Here's how the part is built. I have some questions about the finished solid (model axes, mm). A direction names the side the tool comes from. Give positions to 0.01 mm unless a question says otherwise; leave off trailing zeros. Loops run counter-clockwise (first coordinate to the right, second up) from the corner with the lowest first, then second, coordinate; pieces in that order, holes last. Notation, with made-up numbers: (88.25, -37.75) -> (137.25, -37.75) arc R17 ccw to (137.25, -13.75) -> close; hole circle Ø5 at (19, 78.25). An arc over 180 degrees is marked (long way). Answer in a Markdown table with one row per item. Add a question column.
Item 1: If we section it at C-C (z = 28): Write out the boundary of the cut face in (x, y).
Item 2: For P1, Ø6, axis at x = -107.5, y = 2.5, coming from the +Z side; P2, Ø5, axis at x = 50, y = -3.5, coming from the +Z side; P3, Ø17.5, axis at x = -59.5, z = -14, coming from the +Y side; P4, Ø4, axis at x = 111, y = 5.1, coming from the +Z side, each with a flat end and sliding along its axis, tell me the tip position at first contact or that it passes through.
Item 3: If we section it at B-B (x = -60): Write out the boundary of the cut face in (y, z), then the cut area to 3 significant figures.
Item 4: If we section it at D-D (z = -15): Give the number of separate pieces and of enclosed holes in the cut face, then the cut area to 3 significant figures.
Item 5: We'd pull the mould along Z, two halves only. Please class faces 6 (the face through (-48, -13, -11)), 7 (the face through (110.662, 10.877, 46.735)), 8 (the face through (62.003, -12.714, -14.369)): released by +Z, released by -Z, zero draft, split by the parting line, or undercut.
Item 6: If I drill on line 1 (X direction, y = -10.25, z = 57); line 2 (Z direction, x = 60, y = -15); line 3 (X direction, y = -9.5, z = -16.5), over which ranges is the centre line in solid material (lowest first)?
Item 7: Which directions (+Z, -Z, +X, -X, +Y, -Y) give clear straight access to the entire face, cutting with the end or side of a thin tool? Please do faces 1 (the face through (-107.4, 5, 49)), 2 (the face through (-1, -14.7, 5)), 3 (the face through (-60, -8.7, -10)), 4 (the face through (38, -4, 11.43)), 5 (the face through (62, -13.7, -17)).
Item 8: If we section it at A-A (z = 59): Write out the boundary of the cut face in (x, y).
```python
from build123d import *

# Parameters (mm, degrees)
F1_DEPTH  = 8
F3_DEPTH  = 1.9
F5_DEPTH  = 2.5
F7_DEPTH  = 2.3
F9_W      = 14
F9_H      = 22
F10_DEPTH = 12
F11_DEPTH = 2
F12_W     = 12.1
F12_H     = 20
F13_W     = 12.1
F13_H     = 20
F14_DEPTH = 2
F17_R     = 5.99999
F18_R     = 5.99999
F19_DEPTH = 10
F20_DEPTH = 25
F22_R     = 2.1
F21_R     = 2.1
F23_DEPTH = 10
F24_SIZE  = 1.5
F25_W     = 24
F25_H     = 8
F26_DEPTH = 28
F28_R     = 4.1
F27_R     = 4.1
F29_DEPTH = 3
F30_R     = 2.1
F31_DEPTH = 28.701
F32_R     = 3.6
F33_DEPTH = 3
F34_R     = 5
F35_W     = 20
F35_H     = 8
F36_DEPTH = 5
F37_SIZE  = 1
F38_W     = 27
F38_H     = 8
F39_DEPTH = 2


# Not quite as in the source:
# - a fillet or chamfer is up to 0.001 mm smaller than in the source, because OpenCascade refuses the exact size
# - a feature names something its author has since deleted; it is built from what else it names


with BuildPart() as f1:
    # F0 (on Front) → F1 (new body)
    with BuildSketch(Plane.XZ):
        Polygon((-118.5, 0), (118.5, 0), (118.5, 66.23), (104.5, 66.23), (104.5, 13.43), (-104.5, 13.43), (-104.5, 66.23), (-118.5, 66.23), align=None)
    extrude(amount=F1_DEPTH)

    # F2 (on face) → F3 (join)
    with BuildSketch(Plane.XZ.offset(8)):
        Polygon((-116.6, 66.23), (-118.5, 66.23), (-118.5, 0), (118.5, 0), (118.5, 66.23), (116.6, 66.23), (116.6, 3.43), (-116.6, 3.43), align=None)
    extrude(amount=F3_DEPTH)

    # F4 (on face) → F5 (join)
    with BuildSketch(Plane.XZ.offset(9.9)):
        Polygon((-113.5, 66.23), (-118.5, 66.23), (-118.5, 0), (118.5, 0), (118.5, 66.23), (113.5, 66.23), (113.5, 8), (-113.5, 8), align=None)
    extrude(amount=F5_DEPTH)

    # F6 (on face) → F7 (join)
    with BuildSketch(Plane.XZ.offset(12.4)):
        Polygon((-116.6, 66.23), (-118.5, 66.23), (-118.5, 0), (118.5, 0), (118.5, 66.23), (116.6, 66.23), (116.6, 3.43), (-116.6, 3.43), align=None)
    extrude(amount=F7_DEPTH)

    # F9 (on face) → F10 (join)
    with BuildSketch(Plane(origin=(0, 0, 0), x_dir=(-1, 0, 0), z_dir=(0, 1, 0))):
        with Locations((111.5, 55.23)):
            Rectangle(F9_W, F9_H)
        with Locations((-111.5, 55.23)):
            Rectangle(F9_W, F9_H)
    extrude(amount=F10_DEPTH)

    # F8 (on face) → F11 (join)
    with BuildSketch(Plane.XZ.offset(14.7)):
        Polygon((-111.5, 66.23), (-118.5, 66.23), (-118.5, 0), (118.5, 0), (118.5, 66.23), (111.5, 66.23), (111.5, 7), (-111.5, 7), align=None)
    extrude(amount=F11_DEPTH)

    # F12 (on face) + F13 (on face) → F14 (cut)
    with BuildSketch(Plane.XY.offset(66.23)):
        with Locations((-110.55, 2)):
            Rectangle(F12_W, F12_H)
    with BuildSketch(Plane.XY.offset(66.23)):
        with Locations((110.55, 2)):
            Rectangle(F13_W, F13_H)
    extrude(amount=-F14_DEPTH, mode=Mode.SUBTRACT)

    # F17 (radius 6 in the source; OpenCascade refuses exactly that, so slightly less here)
    f17_edges = [f1.edges().sort_by_distance(p)[0] for p in [
        (-111.5, 0, 44.23),
        (-111.5, 12, 44.23),
    ]]
    fillet(f17_edges, radius=F17_R)

    # F18 (radius 6 in the source; OpenCascade refuses exactly that, so slightly less here)
    f18_edges = [f1.edges().sort_by_distance(p)[0] for p in [
        (111.5, 0, 44.23),
        (111.5, 12, 44.23),
    ]]
    fillet(f18_edges, radius=F18_R)

    # F15 (on face) + F16 (on face) → F19 (cut)
    with BuildSketch(Plane(origin=(0, 0, 44.23), x_dir=(1, 0, 0), z_dir=(0, 0, -1))):
        Polygon((111, -1.1430780618), (107.4, -3.2215390309), (107.4, -7.3784609691), (111, -9.4569219382), (114.6, -7.3784609691), (114.6, -3.2215390309), align=None)
    with BuildSketch(Plane(origin=(0, 0, 44.23), x_dir=(1, 0, 0), z_dir=(0, 0, -1))):
        Polygon((-107.4, -7.3784609691), (-107.4, -3.2215390309), (-111, -1.1430780618), (-114.6, -3.2215390309), (-114.6, -7.3784609691), (-111, -9.4569219382), align=None)
    extrude(amount=-F19_DEPTH, mode=Mode.SUBTRACT)

    # F15 (on face) + F16 (on face) → F20 (cut)
    with BuildSketch(Plane(origin=(0, 0, 44.23), x_dir=(1, 0, 0), z_dir=(0, 0, -1))):
        Polygon((111, -1.1430780618), (107.4, -3.2215390309), (107.4, -7.3784609691), (111, -9.4569219382), (114.6, -7.3784609691), (114.6, -3.2215390309), align=None)
    with BuildSketch(Plane(origin=(0, 0, 44.23), x_dir=(1, 0, 0), z_dir=(0, 0, -1))):
        Polygon((-107.4, -7.3784609691), (-107.4, -3.2215390309), (-111, -1.1430780618), (-114.6, -3.2215390309), (-114.6, -7.3784609691), (-111, -9.4569219382), align=None)
    extrude(amount=F20_DEPTH, mode=Mode.SUBTRACT)

    # F22 (on face) + F21 (on face) → F23 (cut, through all)
    with BuildSketch(Plane.XY.offset(64.23)):
        with Locations((111, 5.1)):
            Circle(F22_R)
    with BuildSketch(Plane.XY.offset(64.23)):
        with Locations((-111, 5.1)):
            Circle(F21_R)
    extrude(amount=-F23_DEPTH, mode=Mode.SUBTRACT)

    # F24
    f24_edges = [f1.edges().sort_by_distance(p)[0] for p in [
        (118.5, 0, 19.115005),
        (-118.5, 0, 19.115005),
        (0, 0, 0),
        (118.5, 12, 58.229995),
        (118.5, 10.242644, 45.987356),
        (118.5, 6, 44.23),
        (118.5, 1.757356, 42.472644),
        (-118.5, 1.757356, 42.472644),
        (-118.5, 6, 44.23),
        (-118.5, 10.242644, 45.987356),
        (-118.5, 12, 58.229995),
    ]]
    chamfer(f24_edges, length=F24_SIZE)

    # F25 (on face) → F26 (join)
    with BuildSketch(Plane(origin=(0, 0, 0), x_dir=(1, 0, 0), z_dir=(0, 0, -1))):
        with Locations((-60, 12.7)):
            Rectangle(F25_W, F25_H)
        with Locations((60, 12.7)):
            Rectangle(F25_W, F25_H)
    extrude(amount=F26_DEPTH)

    # F28 (on face) + F27 (on face) → F29 (cut)
    with BuildSketch(Plane(origin=(0, -8.7, 0), x_dir=(-1, 0, 0), z_dir=(0, 1, 0))):
        with Locations((-60, -15)):
            Circle(F28_R)
    with BuildSketch(Plane(origin=(0, -8.7, 0), x_dir=(-1, 0, 0), z_dir=(0, 1, 0))):
        with Locations((60, -15)):
            Circle(F27_R)
    extrude(amount=-F29_DEPTH, mode=Mode.SUBTRACT)

    # F30 (on face) → F31 (cut, through all)
    with BuildSketch(Plane.XZ.offset(16.7)):
        with Locations((-60, -15)):
            Circle(F30_R)
        with Locations((60, -15)):
            Circle(F30_R)
    extrude(amount=-F31_DEPTH, mode=Mode.SUBTRACT)

    # F32 (on face) → F33 (cut)
    with BuildSketch(Plane.XZ.offset(16.7)):
        with Locations((-60, -15)):
            Circle(F32_R)
        with Locations((60, -15)):
            Circle(F32_R)
    extrude(amount=-F33_DEPTH, mode=Mode.SUBTRACT)

    # F34
    f34_edges = [f1.edges().sort_by_distance(p)[0] for p in [
        (-72, -12.7, -28),
        (-48, -12.7, -28),
        (48, -12.7, -28),
        (72, -12.7, -28),
    ]]
    fillet(f34_edges, radius=F34_R)

    # F35 (on face) → F36 (cut)
    with BuildSketch(Plane.XY.offset(13.43)):
        with Locations((-21.5, -4)):
            Rectangle(F35_W, F35_H)
    extrude(amount=-F36_DEPTH, mode=Mode.SUBTRACT)

    # F37
    f37_edges = [f1.edges().sort_by_distance(p)[0] for p in [
        (-72, -8.7, -11.5),
        (72, -8.7, -11.5),
        (48, -8.7, -11.5),
        (-48, -8.7, -11.5),
        (-70.535534, -8.7, -26.535534),
        (-60, -8.7, -28),
        (-49.464466, -8.7, -26.535534),
        (49.464466, -8.7, -26.535534),
        (60, -8.7, -28),
        (70.535534, -8.7, -26.535534),
    ]]
    chamfer(f37_edges, length=F37_SIZE)

    # F38 (on face) → F39 (cut)
    with BuildSketch(Plane.XY.offset(13.43)):
        with Locations((38.1, -4)):
            Rectangle(F38_W, F38_H)
    extrude(amount=-F39_DEPTH, mode=Mode.SUBTRACT)


solid = f1.part
```
Recorded:
| question | item | result |
|---|---|---|
| 1 | outline | (-118.5, -16.7) -> (-111.5, -16.7) -> (-111.5, -14.7) -> (-116.6, -14.7) -> (-116.6, -12.4) -> (-113.5, -12.4) -> (-113.5, -9.9) -> (-116.6, -9.9) -> (-116.6, -8) -> (-104.5, -8) -> (-104.5, 0) -> (-117, 0) -> (-118.5, -1.5) -> close; (104.5, -8) -> (116.6, -8) -> (116.6, -9.9) -> (113.5, -9.9) -> (113.5, -12.4) -> (116.6, -12.4) -> (116.6, -14.7) -> (111.5, -14.7) -> (111.5, -16.7) -> (118.5, -16.7) -> (118.5, -1.5) -> (117, 0) -> (104.5, 0) -> close |
| 2 | P1 | stops at z = 64.23 |
| 2 | P2 | stops at z = 13.43 |
| 2 | P3 | stops at y = -8.7 |
| 2 | P4 | passes through |
| 3 | outline | (-16.7, -28) -> (-9.7, -28) -> (-8.7, -27) -> (-8.7, -19.1) -> (-11.7, -19.1) -> (-11.7, -17.1) -> (-13.7, -17.1) -> (-13.7, -18.6) -> (-16.7, -18.6) -> close; (-16.7, -11.4) -> (-13.7, -11.4) -> (-13.7, -12.9) -> (-11.7, -12.9) -> (-11.7, -10.9) -> (-8.7, -10.9) -> (-8.7, 0) -> (-1.5, 0) -> (0, 1.5) -> (0, 13.43) -> (-8, 13.43) -> (-8, 3.43) -> (-9.9, 3.43) -> (-9.9, 8) -> (-12.4, 8) -> (-12.4, 3.43) -> (-14.7, 3.43) -> (-14.7, 7) -> (-16.7, 7) -> close |
| 3 | area | 324 mm^2 |
| 4 | separate pieces | 4 |
| 4 | enclosed holes | 0 |
| 4 | area | 273 mm^2 |
| 5 | face 6 | zero draft |
| 5 | face 7 | released by -Z |
| 5 | face 8 | undercut |
| 6 | line 1 | x = -118.5 to -113.5, 113.5 to 118.5 |
| 6 | line 2 | z = -28 to -18.6, -11.4 to 7 |
| 6 | line 3 | x = -71.8 to -63.82, -56.18 to -48.2, 48.2 to 56.18, 63.82 to 71.8 |
| 7 | face 1 | -Z |
| 7 | face 2 | +Z |
| 7 | face 3 | -Z, +X, -X, +Y |
| 7 | face 4 | +Z, +Y, -Y |
| 7 | face 5 | -Y |
| 8 | outline | (-118.5, -16.7) -> (-111.5, -16.7) -> (-111.5, -14.7) -> (-116.6, -14.7) -> (-116.6, -12.4) -> (-113.5, -12.4) -> (-113.5, -9.9) -> (-116.6, -9.9) -> (-116.6, -8) -> (-104.5, -8) -> (-104.5, 12) -> (-117, 12) -> (-118.5, 10.5) -> close; (104.5, -8) -> (116.6, -8) -> (116.6, -9.9) -> (113.5, -9.9) -> (113.5, -12.4) -> (116.6, -12.4) -> (116.6, -14.7) -> (111.5, -14.7) -> (111.5, -16.7) -> (118.5, -16.7) -> (118.5, 10.5) -> (117, 12) -> (104.5, 12) -> close; hole circle Ø4.2 at (-111, 5.1); hole circle Ø4.2 at (111, 5.1) |
